```python
from build123d import *

# Parameters (mm, degrees)
F0_W     = 1346.2
F0_H     = 863.6
F1_DEPTH = 1016
F2_R     = 317.5
F3_DEPTH = 863.6
F4_R     = 685.8
F5_DEPTH = 685.8


with BuildPart() as f1:
    # F0 (on Front) → F1 (new body)
    with BuildSketch(Plane.XZ):
        with Locations((2.302447, 20.795441)):
            Rectangle(F0_W, F0_H)
    extrude(amount=F1_DEPTH)

    # F2 (on face) → F3 (cut)
    with BuildSketch(Plane.XY.offset(452.595441)):
        with Locations((675.402447, -508)):
            Circle(F2_R)
    extrude(amount=-F3_DEPTH, mode=Mode.SUBTRACT)

    # F4 (on face) → F5 (cut)
    with BuildSketch(Plane(origin=(-670.797553, 0, 0), x_dir=(0, -1, 0), z_dir=(-1, 0, 0))):
        with Locations((1016, 452.595441)):
            Circle(F4_R)
    extrude(amount=-F5_DEPTH, mode=Mode.SUBTRACT)


solid = f1.part
```
Check sheet for the modelled part. Datum: model origin and axes. Units: mm. A direction names the side the tool comes from. Give positions to 0.01 mm unless a question says otherwise; leave off trailing zeros. Order: outer loops, then holes, each group sorted by start corner. A loop starts at its lowest first (then second) coordinate and runs counter-clockwise, first axis right, second up. Notation, with made-up numbers: M 0.25,-21.75 L 17.25,-21.75 A31 ccw 17.25,5.25 Z; hole C 85.25,-33 d2. An arc over 180 degrees is marked long. Answer in a Markdown table with one row per item. Add a question column.
Q1. Thickness scan on L1, parallel to Y at x = 590, z = 371; L2, parallel to Y at x = 500, z = -288; L3, parallel to X at y = -661.5, z = 135. Record the ranges inside material, lowest first.
Q2. Sectioned sample at A-A, the plane x = 387. Record the boundary of the cut face in (y, z).
Q3. Release check for a two-part mould opening along Y. For faces 3 (the flat face through (-670.798, -388, -81)), 4 (the cylindrical face through (-332.698, -525.763, -26.977)), 5 (the cylindrical face through (357.98, -501.02, 26.84)) record: released by +Y, released by -Y, zero draft, split by the parting line, or undercut.
Q4. Sectioned sample at D-D, the plane y = -508. Record the boundary of the cut face in (x, z), and give its area (3 significant figures).
Q5. Access from +Z, -Z, +X, -X, +Y, -Y to the whole of each face (thin tool, end or side, straight path). Record for faces 1 (the flat face through (675.402, -919, 15)), 2 (the flat face through (15.002, -744, 191)).
Q6. Gauge pin test, flat ends, axial feed: pin 1 Ø6 at (x, z) = (-209, 243) entering from -Y; pin 2 Ø2 at (y, z) = (-331, 314) entering from +X; pin 3 Ø1 at (y, z) = (-878.5, 364) entering from -X. Record the tip position at first contact, or that the pin passes through.
Q7. Sectioned sample at C-C, the plane x = -150. Record the boundary of the cut face in (y, z).
Q8. Sectioned sample at B-B, the plane z = 147. Record the boundary of the cut face in (x, y).
Verdict:
| question | item | result |
|---|---|---|
| 1 | L1 | -1016 to -813.8, -202.2 to 0 |
| 1 | L2 | -1016 to -772.65, -243.35 to 0 |
| 1 | L3 | 15 to 397.47 |
| 2 | outline | M -1016,-411 L -640.78,-411 L -640.78,452.6 L -1016,452.6 Z; M -375.22,-411 L 0,-411 L 0,452.6 L -375.22,452.6 Z |
| 3 | face 3 | zero draft |
| 3 | face 4 | released by -Y |
| 3 | face 5 | undercut |
| 4 | outline | M -670.8,-411 L 357.9,-411 L 357.9,452.6 L 15,452.6 L 15,-8.12 L -670.8,-8.12 Z |
| 4 | area | 572,000 mm² |
| 5 | face 1 | +Z, -Z, +X, +Y, -Y |
| 5 | face 2 | +Z, -X, -Y |
| 6 | pin 1 | y = -363.98 |
| 6 | pin 2 | x = 412.49 |
| 6 | pin 3 | x = 15 |
| 7 | outline | M -1016,-411 L 0,-411 L 0,452.6 L -330.2,452.6 A685.8 cw -1016,-233.2 Z |
| 8 | outline | M -670.8,-402.05 L 15,-402.05 L 15,-1016 L 675.4,-1016 L 675.4,-825.5 A317.5 cw 675.4,-190.5 L 675.4,0 L -670.8,0 Z |
